Can you work these out from the model? Positions are in its coordinate system, mm. Face numbers are marked on the shaded views. A direction names the side the tool comes from. Coordinates: 2 decimals unless noted, no trailing zeros. Loops run counter-clockwise (first coordinate to the right, second up) from the corner with the lowest first, then second, coordinate; pieces in that order, holes last.
```python
from build123d import *

# Parameters (mm, degrees)
EXTRUDE_1_DEPTH     = 1.5
EXTRUDE_2_DEPTH     = 3
SKETCH_3_R          = 0.6
CUT_EXTRUDE_1_DEPTH = 4
SKETCH_4_R          = 1.55
CUT_EXTRUDE_2_DEPTH = 4
CUT_EXTRUDE_5_DEPTH = 4
SKETCH_9_R          = 12.25
CUT_EXTRUDE_6_DEPTH = 4
EXTRUDE_4_DEPTH     = 3
SKETCH_12_R         = 1.55
EXTRUDE_5_DEPTH     = 3
SKETCH_13_W         = 14
SKETCH_13_H         = 10.026263385
CUT_EXTRUDE_7_DEPTH = 4
SKETCH_14_W         = 3
SKETCH_14_H         = 10.026263385
EXTRUDE_6_DEPTH     = 3
FILLET_1_R          = 1
CHAMFER_1_SIZE      = 1
SKETCH_15_R         = 0.6
CUT_EXTRUDE_8_DEPTH = 4
CUT_EXTRUDE_9_DEPTH = 4
FILLET_2_R          = 0.6


with BuildPart() as part:
    # 草图1 → 凸台-拉伸1 (new body, symmetric)
    with BuildSketch(Plane.XY):
        Polygon((-34.52642222, 8.609923977), (-26.496675247, -8.609923977), (26.496675247, -8.609923977), (34.52642222, 8.609923977), (25.463344349, 12.836106594), (-25.463344349, 12.836106594), align=None)
    extrude(amount=EXTRUDE_1_DEPTH, both=True)

    # 草图2 → 凸台-拉伸2 (add)
    with BuildSketch(Plane.XY.offset(1.5)):
        Polygon((-33.258567434, 5.891000616), (-38.696414157, 3.355291045), (-33.202376754, -8.426710186), (-27.764530032, -5.891000616), (-29.032384817, -3.172077255), (-31.705992789, -4.418801127), (-34.664320621, 1.925353382), (-31.990712649, 3.172077255), align=None)
        Polygon((38.696414157, 3.355291045), (33.202376754, -8.426710186), (27.764530032, -5.891000616), (29.032384817, -3.172077255), (31.705992789, -4.418801127), (34.664320621, 1.925353382), (31.990712649, 3.172077255), (33.258567434, 5.891000616), align=None)
    extrude(amount=-EXTRUDE_2_DEPTH)

    # 草图3 → 切除-拉伸1 (cut, through all)
    with BuildSketch(Plane.XY.offset(1.5)):
        with Locations((-33.512138391, 6.434785288)):
            Circle(SKETCH_3_R)
        with Locations((-34.410749664, 1.38156871)):
            Circle(SKETCH_3_R)
        with Locations((-31.959563746, -3.875016455)):
            Circle(SKETCH_3_R)
        with Locations((-29.285955774, -2.628292582)):
            Circle(SKETCH_3_R)
        with Locations((-31.737141692, 2.628292582)):
            Circle(SKETCH_3_R)
        with Locations((-27.510959075, -6.434785288)):
            Circle(SKETCH_3_R)
        with Locations((27.510959075, -6.434785288)):
            Circle(SKETCH_3_R)
        with Locations((31.737141692, 2.628292582)):
            Circle(SKETCH_3_R)
        with Locations((29.285955774, -2.628292582)):
            Circle(SKETCH_3_R)
        with Locations((31.959563746, -3.875016455)):
            Circle(SKETCH_3_R)
        with Locations((34.410749664, 1.38156871)):
            Circle(SKETCH_3_R)
        with Locations((33.512138391, 6.434785288)):
            Circle(SKETCH_3_R)
    extrude(amount=-CUT_EXTRUDE_1_DEPTH, mode=Mode.SUBTRACT)

    # 草图4 → 切除-拉伸2 (cut, through all)
    with BuildSketch(Plane.XY.offset(1.5)):
        with Locations((-29.875181049, 6.917010638)):
            Circle(SKETCH_4_R)
        with Locations((-24.803761908, -3.958682806)):
            Circle(SKETCH_4_R)
        with Locations((24.803761908, -3.958682806)):
            Circle(SKETCH_4_R)
        with Locations((29.875181049, 6.917010638)):
            Circle(SKETCH_4_R)
    extrude(amount=-CUT_EXTRUDE_2_DEPTH, mode=Mode.SUBTRACT)

    # 草图5 → 切除-拉伸5 (cut, through all)
    with BuildSketch(Plane.XY.offset(1.5)):
        Polygon((-24.798260361, 9.836106594), (-6.847242561, 9.836106594), (-20.846564229, -4.163215074), (-26.914412925, 8.849328448), align=None)
        Polygon((26.914412925, 8.849328448), (20.846564229, -4.163215074), (6.847242561, 9.836106594), (24.798260361, 9.836106594), align=None)
        Polygon((18.050632445, -5.609923977), (-18.050632445, -5.609923977), (-2.604601874, 9.836106594), (2.604601874, 9.836106594), align=None)
    extrude(amount=-CUT_EXTRUDE_5_DEPTH, mode=Mode.SUBTRACT)

    # 草图9 → 切除-拉伸6 (cut, through all)
    with BuildSketch(Plane.XY.offset(1.5)):
        with Locations((0, 11.469324039)):
            Circle(SKETCH_9_R)
    extrude(amount=-CUT_EXTRUDE_6_DEPTH, mode=Mode.SUBTRACT)

    # 草图10 → 凸台-拉伸4 (add)
    with BuildSketch(Plane.XY.offset(1.5)):
        with BuildLine():
            Line((-12.173512453, 12.836106594), (-15.188627504, 12.836106594))
            ThreePointArc((-15.188627504, 12.836106594), (0, -3.780675961), (15.188627504, 12.836106594))
            Line((15.188627504, 12.836106594), (12.173512453, 12.836106594))
            ThreePointArc((12.173512453, 12.836106594), (0, -0.780675961), (-12.173512453, 12.836106594))
        make_face()
    extrude(amount=-EXTRUDE_4_DEPTH)

    # 草图12 → 凸台-拉伸5 (add)
    with BuildSketch(Plane(origin=(0, 0, -1.5), x_dir=(-1, 0, 0), z_dir=(0, 0, -1))):
        with BuildLine():
            Line((-11.457456133, 28.190053348), (-22.208405391, 12.836106594))
            Line((-22.208405391, 12.836106594), (-12.173512453, 12.836106594))
            ThreePointArc((-12.173512453, 12.836106594), (0, 23.719324039), (12.173512453, 12.836106594))
            Line((12.173512453, 12.836106594), (22.208405391, 12.836106594))
            Line((22.208405391, 12.836106594), (11.457456133, 28.190053348))
            ThreePointArc((11.457456133, 28.190053348), (10.38524584, 29.130356539), (9, 29.469324039))
            Line((9, 29.469324039), (-9, 29.469324039))
            ThreePointArc((-9, 29.469324039), (-10.38524584, 29.130356539), (-11.457456133, 28.190053348))
        make_face()
        with Locations((-9, 26.469324039)):
            Circle(SKETCH_12_R, mode=Mode.SUBTRACT)
        with Locations((9, 26.469324039)):
            Circle(SKETCH_12_R, mode=Mode.SUBTRACT)
    extrude(amount=-EXTRUDE_5_DEPTH)

    # 草图13 → 切除-拉伸7 (cut, through all)
    with BuildSketch(Plane(origin=(0, 0, -1.5), x_dir=(-1, 0, 0), z_dir=(0, 0, -1))):
        with Locations((0, -3.596792285)):
            Rectangle(SKETCH_13_W, SKETCH_13_H)
    extrude(amount=-CUT_EXTRUDE_7_DEPTH, mode=Mode.SUBTRACT)

    # 草图14 → 凸台-拉伸6 (add)
    with BuildSketch(Plane(origin=(0, 0, -1.5), x_dir=(-1, 0, 0), z_dir=(0, 0, -1))):
        with Locations((-8.5, -3.596792285)):
            Rectangle(SKETCH_14_W, SKETCH_14_H)
        with Locations((8.5, -3.596792285)):
            Rectangle(SKETCH_14_W, SKETCH_14_H)
    extrude(amount=-EXTRUDE_6_DEPTH)

    # 圆角1
    fillet_1_edges = [part.edges().sort_by_distance(p)[0] for p in [
        (24.798260361, 9.836106594, 0),
        (26.914412925, 8.849328448, 0),
        (20.846564229, -4.163215074, 0),
        (18.050632445, -5.609923977, 0),
        (-18.050632445, -5.609923977, 0),
        (-26.914412925, 8.849328448, 0),
        (-24.798260361, 9.836106594, 0),
        (-20.846564229, -4.163215074, 0),
        (15.162292069, 9.836106594, 0),
        (-15.162292069, 9.836106594, 0),
        (11.258127086, 1.182581381, 0),
        (13.070507936, 3.612841219, 0),
        (-13.070507936, 3.612841219, 0),
        (-11.258127086, 1.182581381, 0),
        (10, -0.044254901, 0),
        (10, -5.609923977, 0),
        (-10, -0.044254901, 0),
        (-10, -5.609923977, 0),
    ]]
    fillet(fillet_1_edges, radius=FILLET_1_R)

    # 倒角1
    chamfer_1_edges = [part.edges().sort_by_distance(p)[0] for p in [
        (-33.202376754, -8.426710186, 0),
        (-38.696414157, 3.355291045, 0),
        (7, -8.609923977, 0),
        (-7, -8.609923977, 0),
        (38.696414157, 3.355291045, 0),
        (33.202376754, -8.426710186, 0),
    ]]
    chamfer(chamfer_1_edges, length=CHAMFER_1_SIZE)

    # 草图15 → 切除-拉伸8 (cut, through all)
    with BuildSketch(Plane.XY.offset(1.5)):
        with Locations((-22.208405391, 13.436106594)):
            Circle(SKETCH_15_R)
        with Locations((22.208405391, 13.436106594)):
            Circle(SKETCH_15_R)
    extrude(amount=-CUT_EXTRUDE_8_DEPTH, mode=Mode.SUBTRACT)

    # 草图16 → 切除-拉伸9 (cut, through all)
    with BuildSketch(Plane.XY.offset(1.5)):
        with BuildLine():
            Line((-18.546081625, 12.836106594), (-15.188627504, 12.836106594))
            ThreePointArc((-15.188627504, 12.836106594), (-14.856302935, 14.912108248), (-14.241610553, 16.922674279))
            ThreePointArc((-14.241610553, 16.922674279), (-14.520472082, 17.66711716), (-15.293427441, 17.481378183))
            Line((-15.293427441, 17.481378183), (-18.546081625, 12.836106594))
        make_face()
        with BuildLine():
            Line((18.546081625, 12.836106594), (15.188627504, 12.836106594))
            ThreePointArc((15.188627504, 12.836106594), (14.856302935, 14.912108248), (14.241610553, 16.922674279))
            ThreePointArc((14.241610553, 16.922674279), (14.520472082, 17.66711716), (15.293427441, 17.481378183))
            Line((15.293427441, 17.481378183), (18.546081625, 12.836106594))
        make_face()
    extrude(amount=-CUT_EXTRUDE_9_DEPTH, mode=Mode.SUBTRACT)

    # 圆角2
    fillet_2_edges = [part.edges().sort_by_distance(p)[0] for p in [
        (-15.188627504, 12.836106594, 0),
        (-18.546081625, 12.836106594, 0),
        (15.188627504, 12.836106594, 0),
        (18.546081625, 12.836106594, 0),
    ]]
    fillet(fillet_2_edges, radius=FILLET_2_R)


solid = part.part
```
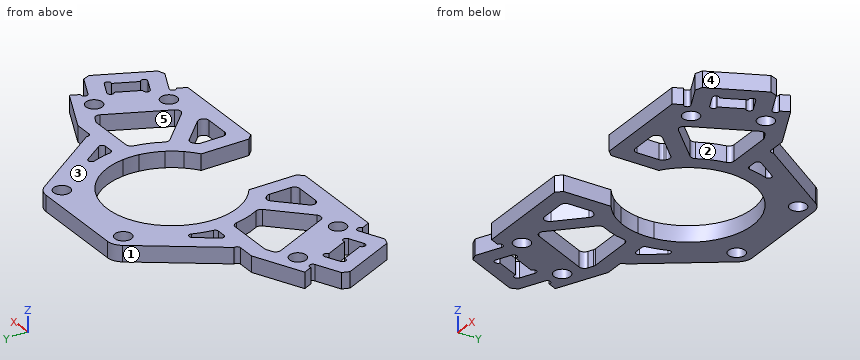
Item 1: Suppose I cut it at D-D, the plane x = 1. Please give me the cut outline in (y, z), plus the area to 3 significant figures.
Results are:
outline: (23.68, -1.5) - (29.47, -1.5) - (29.47, 1.5) - (23.68, 1.5) - close
area: 17.4 mm2
Item 2: On a 3-axis mill with a long thin cutter (end or side, diameter ignored), from which of +Z, -Z, +X, -X, +Y, -Y can I reach the whole of each face in a straight line? I mean the marked faces 1 and 2. Say none if no direction works.
Results are:
face 1: +Z, -Z, -X, +Y
face 2: +Z, -Z
Item 3: We'd pull the mould along X, two halves only. Please class the marked faces 3, 4 and 5: +X half, -X half, draft (parallel to the pull), parting line (faces both ways), or undercut.
Results are:
face 3: draft
face 4: +X half
face 5: undercut
Item 4: I need wall thicknesses on line 1 along Y through (x, z) = (23, 0.6); line 2 along X through (y, z) = (1.5, -0.75); line 3 along X through (y, z) = (15, 1.2). Which ranges of each line are inside material? Lowest first, please.
Results are:
line 1: y = -8.61 to 0.45, 9.84 to 12.84
line 2: x = -37.83 to -35, -31.21 to -23.49, -15.18 to -7.12, 7.12 to 15.18, 23.49 to 31.21, 35 to 37.83
line 3: x = -20.69 to -17.03, -14.84 to -11.73, 11.73 to 14.84, 17.03 to 20.69
Item 5: Suppose I cut it at C-C, the plane z = -0.95. Count the separate pieces of the cut face and the enclosed holes in it, plus the area to 3 significant figures.
Results are:
separate pieces: 1
enclosed holes: 14
area: 1,010 mm2
Item 6: I'm going to push flat-ended pins straight in: P1, Ø1.8, axis at x = -16.5, z = -0.5, coming from the +Y side; P2, Ø0.9, axis at x = -14, z = 0.5, coming from the +Y side. Where does each tip first touch, or does it pass through?
Results are:
P1: stops at y = 22.27
P2: stops at y = 25.2
Item 7: Suppose I cut it at B-B, the plane y = 12. Please give me the cut outline in (x, z).
Results are:
outline: (-27.26, -1.5) - (-12.24, -1.5) - (-12.24, 1.5) - (-27.26, 1.5) - close; (12.24, -1.5) - (27.26, -1.5) - (27.26, 1.5) - (12.24, 1.5) - close
Item 8: Suppose I cut it at A-A, the plane y = 16. Please give me the cut outline in (x, z).
Results are:
outline: (-19.99, -1.5) - (-16.33, -1.5) - (-16.33, 1.5) - (-19.99, 1.5) - close; (-14.56, -1.5) - (-11.38, -1.5) - (-11.38, 1.5) - (-14.56, 1.5) - close; (11.38, -1.5) - (14.56, -1.5) - (14.56, 1.5) - (11.38, 1.5) - close; (16.33, -1.5) - (19.99, -1.5) - (19.99, 1.5) - (16.33, 1.5) - close
